The listing builds one solid part. Answer for the finished solid, in the listing's coordinates (mm). A direction names the side the tool comes from. Coordinates: 2 decimals unless noted, no trailing zeros. Loops run counter-clockwise (first coordinate to the right, second up) from the corner with the lowest first, then second, coordinate; pieces in that order, holes last. Notation, with made-up numbers: M 21.5,16.25 L 32.5,16.25 A23 ccw 32.5,41.25 Z; hole C 59,-15 d9. An arc over 180 degrees is marked long. Answer as a JSON object with one key per item and string values. Group by question number.
1. A cutting plane is placed at C-C on z = 66.5. Give the vertices of the cut face in (x, y).
2. For faces 1 (the face through (-92, -75, 76.2)), 2 (the face through (-141, -152.4, 60)), determine the directions among +Z, -Z, +X, -X, +Y, -Y from which every point of the face is accessible in a straight line to the end or side of a thin tool.
3. A cutting plane is placed at D-D on y = -46. Give the vertices of the cut face in (x, z), and give its area (3 significant figures).
4. A cutting plane is placed at B-B on y = -76.2. Give the vertices of the cut face in (x, z), and give its area (3 significant figures).
5. Determine the mould class of faces 3 (the face through (-30.643, -91.656, 37.567)), 4 (the face through (-228.6, -75, 77)), 5 (the face through (-190, -75, 152.4)), 6 (the face through (0, -75, 38)) for opening direction X: released by +X, released by -X, zero draft, split by the parting line, or undercut.
6. Straight lines are drawn through the part: L1, parallel to X at y = -76, z = 41; L2, parallel to Y at x = -50, z = 56; L3, parallel to Z at x = -45, y = -34. For each, find the intervals that lie inside material, in ascending order.
7. A cutting plane is placed at A-A on x = -50.8. Give the vertices of the cut face in (y, z), and give its area (3 significant figures).
8. Given pin 1 (23 mm diameter, centred on y = -61.5, z = 128, fed in from +X), flat-ended and moving along its own axis, determine where the tip first touches the part or whether it passes through.
from build123d import *

# Parameters (mm, degrees)
F1_DEPTH = 152.4
F3_D     = 50.8


with BuildPart() as f1:
    # F0 (on Front) → F1 (new body)
    with BuildSketch(Plane.XZ):
        Polygon((-228.6, 0), (0, 0), (0, 76.2), (-152.4, 76.2), (-152.4, 152.4), (-228.6, 152.4), align=None)
    extrude(amount=F1_DEPTH)

    # F3 (through all)
    with Locations(Plane.XY.offset(76.2)):
        with Locations((-50.8, -76.2)):
            Hole(F3_D / 2)


solid = f1.part
From the geometry:
{
 "1": {"outline": "M -228.6,-152.4 L 0,-152.4 L 0,0 L -228.6,0 Z; hole C -50.8,-76.2 d50.8"},
 "2": {"face 1": "+Z, +X, +Y, -Y", "face 2": "+Z, -Z, +X, -X, -Y"},
 "3": {"outline": "M -228.6,0 L 0,0 L 0,76.2 L -152.4,76.2 L -152.4,152.4 L -228.6,152.4 Z", "area": "23,200 mm²"},
 "4": {"outline": "M -228.6,0 L -76.2,0 L -76.2,76.2 L -152.4,76.2 L -152.4,152.4 L -228.6,152.4 Z; M -25.4,0 L 0,0 L 0,76.2 L -25.4,76.2 Z", "area": "19,400 mm²"},
 "5": {"face 3": "undercut", "face 4": "released by -X", "face 5": "zero draft", "face 6": "released by +X"},
 "6": {"L1": "x = -228.6 to -76.2, -25.4 to 0", "L2": "y = -152.4 to -101.59, -50.81 to 0", "L3": "z = 0 to 76.2"},
 "7": {"outline": "M -152.4,0 L -101.6,0 L -101.6,76.2 L -152.4,76.2 Z; M -50.8,0 L 0,0 L 0,76.2 L -50.8,76.2 Z", "area": "7,740 mm²"},
 "8": {"pin 1": "stops at x = -152.4"}
}
